Could you check a few things on this model? Use its own coordinates, in mm. Face numbers are marked on the shaded views. Give positions to 0.01 mm unless a question says otherwise; leave off trailing zeros. Loops run counter-clockwise (first coordinate to the right, second up) from the corner with the lowest first, then second, coordinate; pieces in that order, holes last. Notation, with made-up numbers: M 39.25,29 L 75.25,29 A25 cw 75.25,61 Z; hole C 3.25,28 d1. An arc over 180 degrees is marked long. Use a Markdown table: item, result. Add a question column.
1) Suppose I cut it at D-D on y = 4.25. List the corners of the cut face in (x, z) for me, and give its area (3 significant figures).
2) Suppose I cut it at A-A on x = 0. List the corners of the cut face in (y, z) for me.
3) We'd pull the mould along X, two halves only. Please class the marked faces 1, 2 and 3: +X half, -X half, draft (parallel to the pull), parting line (faces both ways), or undercut.
4) Suppose I cut it at C-C on z = 2.25. List the corners of the cut face in (x, y) for me.
5) Will these pins go through, and if not, where does the flat tip stop? pin 1 Ø0.8 at (x, y) = (3.5, -3.5) entering from -Z; pin 2 Ø1.5 at (y, z) = (3, 2) entering from -X; pin 3 Ø0.9 at (y, z) = (-4, 2) entering from +X.
6) If I drill on line 1 along Y through (x, z) = (0, 3.65); line 2 along Y through (x, z) = (5, 1.8), over which ranges is the centre line in solid material (lowest first)? Write a range as [from, to].
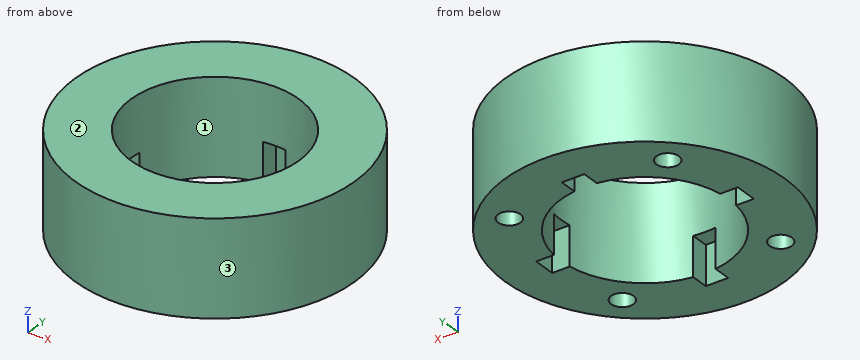
```python
from build123d import *
from build123d.topology import SkipClean

# Parameters (mm, degrees)
SKETCH1_R               = 6.25
SKETCH1_R_2             = 3.75
BOSS_EXTRUDE1_DEPTH     = 5
BOSS_EXTRUDE2_START     = 3
SKETCH2_R               = 5.5
SKETCH2_R_2             = 3.75
BOSS_EXTRUDE2_DEPTH     = 3
THREAD1_PITCH           = 0.6
BOSS_EXTRUDE3_START     = 1.25
SKETCH7_R               = 5
SKETCH7_R_2             = 3.75
BOSS_EXTRUDE3_DEPTH     = 1.25
CUT_EXTRUDE3_DEPTH      = 6.5
CUT_EXTRUDE3_DEPTH_BACK = 5.5
SKETCH5_W               = 1
SKETCH5_H               = 1
BOSS_EXTRUDE4_START     = 0.5
SKETCH8_R               = 5
SKETCH8_R_2             = 3
BOSS_EXTRUDE4_DEPTH     = 0.5
CUT_EXTRUDE4_DEPTH      = 10
CUT_EXTRUDE4_DEPTH_BACK = 10
SKETCH9_W               = 18.419335543
SKETCH9_H               = 5.81075095
SKETCH10_R              = 0.5
CUT_EXTRUDE5_DEPTH      = 2.5
CIRPATTERN1_COUNT       = 4


with BuildPart() as part:
    # Sketch1 → Boss-Extrude1 (new body)
    with BuildSketch(Plane.XY):
        Circle(SKETCH1_R)
        Circle(SKETCH1_R_2, mode=Mode.SUBTRACT)
    extrude(amount=BOSS_EXTRUDE1_DEPTH)

    # Sketch2 → Boss-Extrude2 (add)
    with SkipClean():  # the faces are left unmerged after this step: merging them gives an invalid solid
        with BuildSketch(Plane(origin=(0, 0, 0), x_dir=(-1, 0, 0), z_dir=(0, 0, -1)).offset(BOSS_EXTRUDE2_START)):
            Circle(SKETCH2_R)
            Circle(SKETCH2_R_2, mode=Mode.SUBTRACT)
        extrude(amount=-BOSS_EXTRUDE2_DEPTH)

    # Thread1: the profile of Thread Profile1 profile screwed along a right-hand helix of 6.666667 turns, 6 arcs to a turn; built about Z, then put on its axis
    with SkipClean():  # the faces are left unmerged after this step: merging them gives an invalid solid
        thread1_z = Axis((0, 0, 0), (0, 0, 1))
        thread1_corners = [(5.5003, 0, -0.000173205), (5.5003, 0, 0.525173203), (5.175240475, 0, 0.337499999), (5.175240475, 0, 0.187499999)]
        with BuildLine(mode=Mode.PRIVATE) as thread1_profile:
            Line(thread1_corners[0], thread1_corners[1])
            Line(thread1_corners[1], thread1_corners[2])
            Line(thread1_corners[2], thread1_corners[3])
            Line(thread1_corners[3], thread1_corners[0])
        thread1_cap = Face(thread1_profile.wire())
        thread1_turn_angles = [0, 30, 60, 90, 120, 150, 180, 210, 240, 270, 300, 330, 360]
        thread1_turn_weights = [1, 0.8660254037844387, 1, 0.8660254037844387, 1, 0.8660254037844387, 1, 0.8660254037844387, 1, 0.8660254037844387, 1, 0.8660254037844387, 1]
        thread1_turn_rails = [Edge.make_bspline([Vector(p[0], p[1], 0).rotate(thread1_z, thread1_turn_angles[k]) / thread1_turn_weights[k] + Vector(0, 0, p[2] + THREAD1_PITCH * thread1_turn_angles[k] / 360) for k in range(13)], [0, 0, 0, 1, 1, 2, 2, 3, 3, 4, 4, 5, 5, 6, 6, 6], 2, thread1_turn_weights) for p in thread1_corners]
        thread1_turn_sides = [Face.make_surface_from_curves(thread1_turn_rails[p[0]], thread1_turn_rails[p[1]]) for p in [(0, 1), (1, 2), (2, 3), (3, 0)]]
        thread1_last_angles = [2160, 2190, 2220, 2250, 2280, 2310, 2340, 2370, 2400]
        thread1_last_weights = [1, 0.8660254037844387, 1, 0.8660254037844387, 1, 0.8660254037844387, 1, 0.8660254037844387, 1]
        thread1_last_rails = [Edge.make_bspline([Vector(p[0], p[1], 0).rotate(thread1_z, thread1_last_angles[k]) / thread1_last_weights[k] + Vector(0, 0, p[2] + THREAD1_PITCH * thread1_last_angles[k] / 360) for k in range(9)], [0, 0, 0, 1, 1, 2, 2, 3, 3, 4, 4, 4], 2, thread1_last_weights) for p in thread1_corners]
        thread1_last_sides = [Face.make_surface_from_curves(thread1_last_rails[p[0]], thread1_last_rails[p[1]]) for p in [(0, 1), (1, 2), (2, 3), (3, 0)]]
        thread1 = Plane(origin=(0, 0, -4), x_dir=(1, 0, 0), z_dir=(0, 0, 1)) * Solid(Shell([*[p.moved(Location((0, 0, THREAD1_PITCH * i))) for i in range(6) for p in thread1_turn_sides], *thread1_last_sides, thread1_cap, thread1_cap.rotate(thread1_z, 2400).moved(Location((0, 0, THREAD1_PITCH * 2400 / 360)))]))
        add(thread1, mode=Mode.SUBTRACT)

    # Sketch7 → Boss-Extrude3 (add)
    with SkipClean():  # the faces are left unmerged after this step: merging them gives an invalid solid
        with BuildSketch(Plane(origin=(0, 0, -3), x_dir=(-1, 0, 0), z_dir=(0, 0, -1)).offset(BOSS_EXTRUDE3_START)):
            Circle(SKETCH7_R)
            Circle(SKETCH7_R_2, mode=Mode.SUBTRACT)
        extrude(amount=-BOSS_EXTRUDE3_DEPTH)

    # Sketch5 → Cut-Extrude3 (cut, two sides: drawn at the far end of the back side and taken through both)
    with BuildSketch(Plane(origin=(0, 0, -3), x_dir=(-1, 0, 0), z_dir=(0, 0, -1)).offset(-CUT_EXTRUDE3_DEPTH_BACK)):
        with Locations((4, 0)):
            Rectangle(SKETCH5_W, SKETCH5_H)
        with Locations((0, 4)):
            Rectangle(SKETCH5_W, SKETCH5_H)
        with Locations((0, -4)):
            Rectangle(SKETCH5_W, SKETCH5_H)
        with Locations((-4, 0)):
            Rectangle(SKETCH5_W, SKETCH5_H)
    extrude(amount=CUT_EXTRUDE3_DEPTH + CUT_EXTRUDE3_DEPTH_BACK, mode=Mode.SUBTRACT)

    # Sketch8 → Boss-Extrude4 (add)
    with BuildSketch(Plane(origin=(0, 0, -4.25), x_dir=(-1, 0, 0), z_dir=(0, 0, -1)).offset(BOSS_EXTRUDE4_START)):
        Circle(SKETCH8_R)
        Circle(SKETCH8_R_2, mode=Mode.SUBTRACT)
    extrude(amount=-BOSS_EXTRUDE4_DEPTH)

    # Sketch9 → Cut-Extrude4 (cut, two sides: drawn at the far end of the back side and taken through both)
    with BuildSketch(Plane(origin=(0, 0, 0), x_dir=(1, 0, 0), z_dir=(0, 1, 0)).offset(-CUT_EXTRUDE4_DEPTH_BACK)):
        with Locations((-0.0093121, 2.155375475)):
            Rectangle(SKETCH9_W, SKETCH9_H)
    extrude(amount=CUT_EXTRUDE4_DEPTH + CUT_EXTRUDE4_DEPTH_BACK, mode=Mode.SUBTRACT)

    # Sketch10 → Cut-Extrude5 (cut)
    with BuildSketch(Plane(origin=(0, 0, 0.75), x_dir=(-1, 0, 0), z_dir=(0, 0, -1))):
        with Locations((-3.535533906, 3.535533906)):
            Circle(SKETCH10_R)
    cut_extrude5 = extrude(amount=-CUT_EXTRUDE5_DEPTH, mode=Mode.SUBTRACT)

    # CirPattern1: Cut-Extrude5 ×4 about axis
    cirpattern1_axis = Axis((0, 0, 0), (0, 0, 1))
    for i in range(1, CIRPATTERN1_COUNT):
        add(cut_extrude5.rotate(cirpattern1_axis, i * 360 / CIRPATTERN1_COUNT), mode=Mode.SUBTRACT)


solid = part.part
```
Answer block:
| question | item | result |
|---|---|---|
| 1 | outline | M -4.58,0.75 L -0.5,0.75 L -0.5,2.5 L 0.5,2.5 L 0.5,0.75 L 4.58,0.75 L 4.58,5 L -4.58,5 Z |
| 1 | area | 37.2 mm^2 |
| 2 | outline | M -6.25,0.75 L -4.5,0.75 L -4.5,2.5 L -3.75,2.5 L -3.75,5 L -6.25,5 Z; M 3.75,2.5 L 4.5,2.5 L 4.5,0.75 L 6.25,0.75 L 6.25,5 L 3.75,5 Z |
| 3 | face 1 | undercut |
| 3 | face 2 | draft |
| 3 | face 3 | parting line |
| 4 | outline | C 0,0 d12.5; hole M -4.5,-0.5 L -3.72,-0.5 A3.75 ccw -0.5,-3.72 L -0.5,-4.5 L 0.5,-4.5 L 0.5,-3.72 A3.75 ccw 3.72,-0.5 L 4.5,-0.5 L 4.5,0.5 L 3.72,0.5 A3.75 ccw 0.5,3.72 L 0.5,4.5 L -0.5,4.5 L -0.5,3.72 A3.75 ccw -3.72,0.5 L -4.5,0.5 Z; hole C -3.54,-3.54 d1; hole C -3.54,3.54 d1; hole C 3.54,-3.54 d1; hole C 3.54,3.54 d1 |
| 5 | pin 1 | stops at z = 3.25 |
| 5 | pin 2 | stops at x = -5.83 |
| 5 | pin 3 | stops at x = 5.14 |
| 6 | line 1 | y = [-6.25, -3.75], [3.75, 6.25] |
| 6 | line 2 | y = [-3.75, 3.75] |
